The model under review builds one solid part; all positions refer to its coordinate system, in mm. Coordinates: 2 decimals unless noted, no trailing zeros. Write each loop counter-clockwise with the first axis right and the second up, starting at its lowest first coordinate (ties: lowest second). Pieces come first, ordered by that corner, then holes. Notation, with made-up numbers: (-37.75, -36.5) -> (-11.75, -36.5) arc R27 ccw to (-11.75, -8.5) -> close; hole circle Ø5 at (-30.75, 40). An arc over 180 degrees is marked (long way). Write each question's results on one line, items separated by ' | '.
```python
from build123d import *

# Parameters (mm, degrees)
SKETCH_1_W                  = 200
SKETCH_1_H                  = 320
EXTRUDE_1_DEPTH             = 12
HOLE_WIZARD_2_D             = 8.5
HOLE_WIZARD_2_CBORE_D       = 13
HOLE_WIZARD_2_CBORE_DEPTH   = 8.5
CHAMFER_1_SIZE              = 10
SKETCH_4_R                  = 11.25
CUT_EXTRUDE_1_DEPTH         = 190.06083677
HOLE_WIZARD_2_2_D           = 6.5
HOLE_WIZARD_2_2_CBORE_D     = 11
HOLE_WIZARD_2_2_CBORE_DEPTH = 6.5
SKETCH_7_R                  = 24.25
CUT_EXTRUDE_2_DEPTH         = 6
SKETCH_8_R                  = 14.25
CUT_EXTRUDE_3_DEPTH         = 189.774998345
HOLE_WIZARD_M4_1_D          = 3.3


with BuildPart() as part:
    # 草图1 → 凸台-拉伸1 (new body)
    with BuildSketch(Plane(origin=(0, 0, 0), x_dir=(1, 0, 0), z_dir=(0, 1, 0))):
        Rectangle(SKETCH_1_W, SKETCH_1_H)
    extrude(amount=EXTRUDE_1_DEPTH)

    # Hole Wizard 2 (through all)
    with Locations(Plane(origin=(0, 12, 0), x_dir=(1, 0, 0), z_dir=(0, 1, 0))):
        with Locations((-75, 140), (75, 140), (75, -140), (-75, -140), (0, 140), (0, -140)):
            CounterBoreHole(HOLE_WIZARD_2_D / 2, HOLE_WIZARD_2_CBORE_D / 2, HOLE_WIZARD_2_CBORE_DEPTH)

    # 倒角1
    chamfer_1_edges = [part.edges().sort_by_distance(p)[0] for p in [
        (100, 6, 160),
        (-100, 6, 160),
        (-100, 6, -160),
        (100, 6, -160),
    ]]
    chamfer(chamfer_1_edges, length=CHAMFER_1_SIZE)

    # 草图4 → 切除-拉伸1 (cut, through all)
    with BuildSketch(Plane(origin=(0, 0, 0), x_dir=(-1, 0, 0), z_dir=(0, -1, 0))):
        with Locations(Location((0, 0, 0), (0, 0, 90))):
            Circle(SKETCH_4_R)
    extrude(amount=-CUT_EXTRUDE_1_DEPTH, mode=Mode.SUBTRACT)

    # Hole Wizard 2 2 (through all)
    with Locations(Plane(origin=(0, 12, 0), x_dir=(1, 0, 0), z_dir=(0, 1, 0))):
        with Locations((-17, 17), (-17, -17), (17, -17), (17, 17)):
            CounterBoreHole(HOLE_WIZARD_2_2_D / 2, HOLE_WIZARD_2_2_CBORE_D / 2, HOLE_WIZARD_2_2_CBORE_DEPTH)

    # 草图7 → 切除-拉伸2 (cut)
    with BuildSketch(Plane(origin=(0, 12, 0), x_dir=(1, 0, 0), z_dir=(0, 1, 0))):
        with Locations(Location((-70, 0, 0), (0, 0, 270))):
            Circle(SKETCH_7_R)
        with Locations(Location((70, 0, 0), (0, 0, 90))):
            Circle(SKETCH_7_R)
    extrude(amount=-CUT_EXTRUDE_2_DEPTH, mode=Mode.SUBTRACT)

    # 草图8 → 切除-拉伸3 (cut, through all)
    with BuildSketch(Plane(origin=(0, 6, 0), x_dir=(1, 0, 0), z_dir=(0, 1, 0))):
        with Locations(Location((-70, 0, 0), (0, 0, 270))):
            Circle(SKETCH_8_R)
        with Locations(Location((70, 0, 0), (0, 0, 90))):
            Circle(SKETCH_8_R)
    extrude(amount=-CUT_EXTRUDE_3_DEPTH, mode=Mode.SUBTRACT)

    # M4 螺纹孔1 (through all)
    with Locations(Plane(origin=(0, 12, 0), x_dir=(1, 0, 0), z_dir=(0, 1, 0))):
        with Locations((-70, 19), (-89, 0), (-70, -19), (-51, 0), (51, 0), (70, -19), (89, 0), (70, 19)):
            Hole(HOLE_WIZARD_M4_1_D / 2)


solid = part.part
```
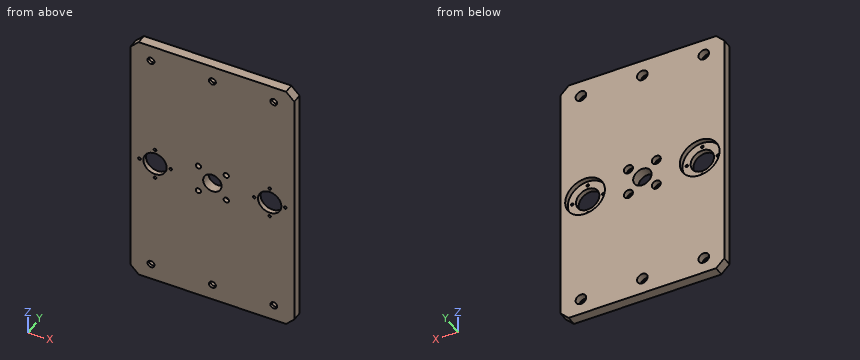
Q1. Clearance check with flat-ended pins moving along their axes: P1, Ø4, axis at x = -78, z = 143, coming from the +Y side; P2, Ø14.5, axis at x = 59.5, z = 6.5, coming from the +Y side; P3, Ø10.5, axis at x = 17, z = 17, coming from the +Y side. State where each tip first meets the part, or that it passes through.
Solution:
P1: y = 3.5 | P2: y = 6 | P3: y = 5.5
Q2. For line 1 (X direction, y = 7.75, z = 140); line 2 (X direction, y = 8.6, z = 0); line 3 (X direction, y = 9.75, z = -17), list the stretches that pass through material, from the lowest coordinate up. Write a range as from..to.
Solution:
line 1: -100..-81.5, -68.5..-6.5, 6.5..68.5, 81.5..100 | line 2: -100..-94.25, -45.75..-11.25, 11.25..45.75, 94.25..100 | line 3: -100..-87.29, -52.71..-22.5, -11.5..11.5, 22.5..52.71, 87.29..100
Q3. Add section A-A (z = 140). Write out the cut boundary in (x, y).
Solution:
outline: (-100, 0) -> (-79.25, 0) -> (-79.25, 3.5) -> (-81.5, 3.5) -> (-81.5, 12) -> (-100, 12) -> close; (-70.75, 0) -> (-4.25, 0) -> (-4.25, 3.5) -> (-6.5, 3.5) -> (-6.5, 12) -> (-68.5, 12) -> (-68.5, 3.5) -> (-70.75, 3.5) -> close; (4.25, 0) -> (70.75, 0) -> (70.75, 3.5) -> (68.5, 3.5) -> (68.5, 12) -> (6.5, 12) -> (6.5, 3.5) -> (4.25, 3.5) -> close; (79.25, 0) -> (100, 0) -> (100, 12) -> (81.5, 12) -> (81.5, 3.5) -> (79.25, 3.5) -> close
Q4. Add section B-B (x = 17). Write out the cut boundary in (y, z).
Solution:
outline: (0, -160) -> (12, -160) -> (12, -22.5) -> (5.5, -22.5) -> (5.5, -20.25) -> (0, -20.25) -> close; (0, -13.75) -> (5.5, -13.75) -> (5.5, -11.5) -> (12, -11.5) -> (12, 11.5) -> (5.5, 11.5) -> (5.5, 13.75) -> (0, 13.75) -> close; (0, 20.25) -> (5.5, 20.25) -> (5.5, 22.5) -> (12, 22.5) -> (12, 160) -> (0, 160) -> close
